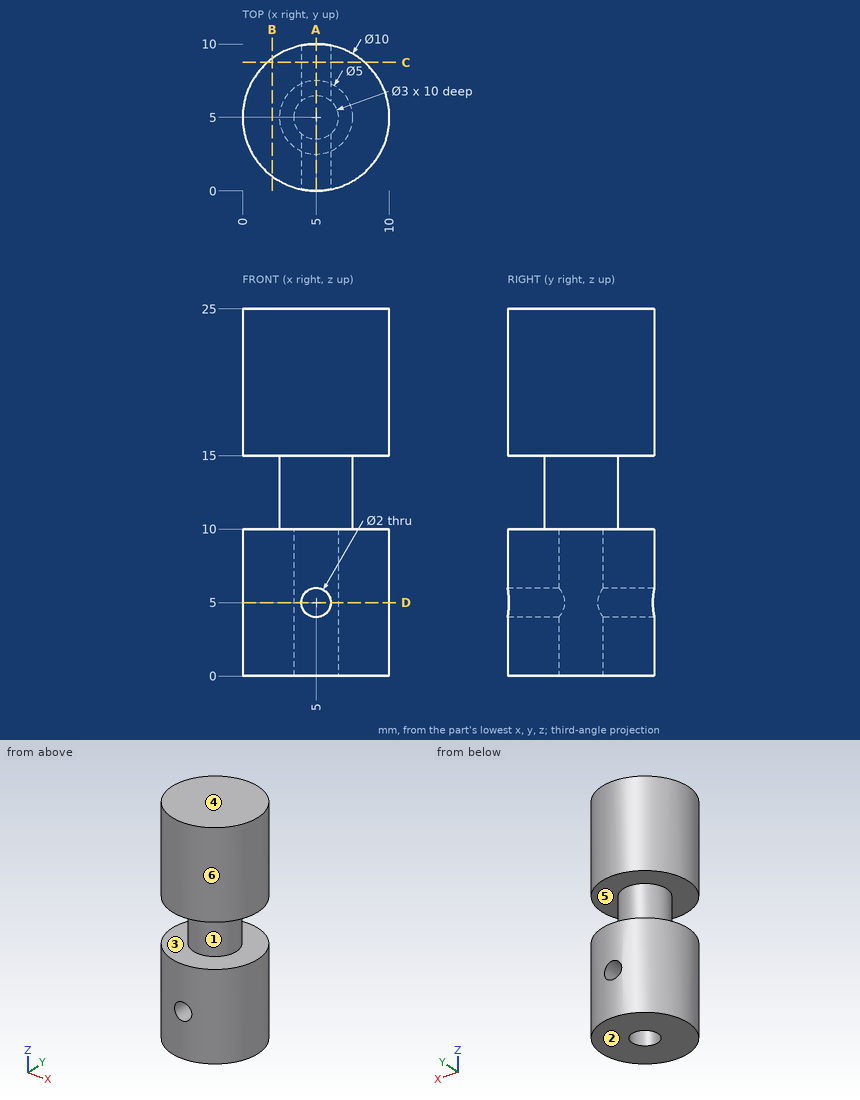
The figure shows three views and two pictorial views of one solid part (mm, origin at its lowest corner). Answer the questions. A direction names the side the tool comes from. Coordinates: 2 decimals unless noted, no trailing zeros. Loops run counter-clockwise (first coordinate to the right, second up) from the corner with the lowest first, then second, coordinate; pieces in that order, holes last.
1) Find section D-D on z = 5. Write down the section's boundary in (x, y), then the cut area to 3 significant figures.
2) Find the intervals of material crossed by L1, parallel to Z at x = 8, y = 2; L2, parallel to X at y = 2.85, z = 5; L3, parallel to X at y = 4.5, z = 6.75, in increasing order.
3) Find section B-B on x = 2. Write down the section's boundary in (y, z).
4) Flat-ended cylindrical pins translate along their axes: pin 1 Ø2 at (y, z) = (8.5, 20) entering from +X; pin 2 Ø1 at (y, z) = (3.5, 15.5) entering from -X; pin 3 Ø1.5 at (x, z) = (1, 7.5) entering from +Y. Find the tip coordinate at first contact, or state that the pin passes through.
5) A tool of negligible diameter and unlimited length cuts with its end or side. For the marked faces 1 and 2, from which of +Z, -Z, +X, -X, +Y, -Y can it reach the whole face along a straight path? Write none if from no direction.
6) Find section A-A on x = 5. Write down the section's boundary in (y, z), then the cut area to 3 significant figures.
7) Determine the mould class of the marked faces 3, 4, 5 and 6 for opening direction Z: pulls with the +Z half, pulls with the -Z half, needs draft (parallel to the pull), parting line crosses it, or undercut.
8) Find section C-C on y = 8.75. Write down the section's boundary in (x, z), then the cut area to 3 significant figures.
Values:
1. outline: (4, 0.1) - (4, 3.88) arc R1.5 cw to (4, 6.12) - (4, 9.9) arc R5 ccw to start; (6, 0.1) arc R5 ccw to (6, 9.9) - (6, 6.12) arc R1.5 cw to (6, 3.88) - close
1. area: 57.1 mm2
2. L1: z = 0 to 10, 15 to 25
2. L2: x = 0.49 to 4, 6 to 9.51
2. L3: x = 0.03 to 3.59, 6.41 to 9.97
3. outline: (1, 0) - (9, 0) - (9, 10) - (1, 10) - close; (1, 15) - (9, 15) - (9, 25) - (1, 25) - close
4. pin 1: stops at x = 9.33
4. pin 2: stops at x = 0.1
4. pin 3: stops at y = 8.8
5. face 1: none
5. face 2: -Z, +X, -X, +Y, -Y
6. outline: (0, 0) - (3.5, 0) - (3.5, 4) - (0, 4) - close; (0, 6) - (3.5, 6) - (3.5, 10) - (6.5, 10) - (6.5, 6) - (10, 6) - (10, 10) - (7.5, 10) - (7.5, 15) - (10, 15) - (10, 25) - (0, 25) - (0, 15) - (2.5, 15) - (2.5, 10) - (0, 10) - close; (6.5, 0) - (10, 0) - (10, 4) - (6.5, 4) - close
6. area: 181 mm2
7. face 3: undercut
7. face 4: pulls with the +Z half
7. face 5: undercut
7. face 6: needs draft
8. outline: (1.69, 0) - (8.31, 0) - (8.31, 10) - (1.69, 10) - close; (1.69, 15) - (8.31, 15) - (8.31, 25) - (1.69, 25) - close; hole circle Ø2 at (5, 5)
8. area: 129 mm2
